from build123d import *

# Parameters (mm, degrees)
ESQUISSE1_W             = 260
ESQUISSE1_H             = 450
BOSS_EXTRU_1_DEPTH      = 130.18
ENL_V_MAT_EXTRU_1_REACH = 488.155
ESQUISSE2_W             = 240
ESQUISSE2_H             = 240.36


with BuildPart() as part:
    # Esquisse1 → Boss.-Extru.1 (new, symmetric)
    with BuildSketch(Plane.XY):
        Rectangle(ESQUISSE1_W, ESQUISSE1_H)
    extrude(amount=BOSS_EXTRU_1_DEPTH, both=True)

    # Esquisse2 → Enlèv. mat.-Extru.1 (cut, up to next)
    with BuildSketch(Plane(origin=(0, 225, 0), x_dir=(1, 0, 0), z_dir=(0, 1, 0)), mode=Mode.PRIVATE) as enl_v_mat_extru_1_sk1:
        Rectangle(ESQUISSE2_W, ESQUISSE2_H)
    enl_v_mat_extru_1_tool1 = extrude(enl_v_mat_extru_1_sk1.sketch, amount=-ENL_V_MAT_EXTRU_1_REACH, mode=Mode.PRIVATE) & part.part
    add(enl_v_mat_extru_1_tool1.solids().sort_by_distance((0, 225, 0))[0], mode=Mode.SUBTRACT)


solid = part.part
Here's how the part is built. I have some questions about the finished solid (model axes, mm). A direction names the side the tool comes from. Give positions to 0.01 mm unless a question says otherwise; leave off trailing zeros. Order: outer loops, then holes, each group sorted by start corner. A loop starts at its lowest first (then second) coordinate and runs counter-clockwise, first axis right, second up. Notation, with made-up numbers: M 88,-20.5 L 106,-20.5 A21 cw 106,-11.5 Z; hole C 41,54.5 d7. An arc over 180 degrees is marked long. Answer as a JSON object with one key per item and string values. Group by question number.
1) We'd pull the mould along Z, two halves only. Please class faces 3 (the flat face through (-2, 3, -120.18)), 4 (the flat face through (-2, 3, 130.18)), 5 (the flat face through (-10, -225, -125)): pulls with the +Z half, pulls with the -Z half, needs draft (parallel to the pull), parting line crosses it, or undercut.
2) Suppose I cut it at C-C, the plane y = -35.5. Write out the boundary of the cut face in (x, z).
3) Please list where these lines run through material, in increasing order: L1, parallel to Z at x = -3, y = -81.5; L2, parallel to X at y = 181, z = 78. Write a range as [from, to].
4) Suppose I cut it at A-A, the plane x = -77.5. Write out the boundary of the cut face in (y, z).
5) Suppose I cut it at B-B, the plane z = 79. Write out the boundary of the cut face in (x, y), plus the area to 3 significant figures.
6) On a 3-axis mill with a long thin cutter (end or side, diameter ignored), from which of +Z, -Z, +X, -X, +Y, -Y can I reach the whole of each face in a straight line? I mean faces 1 (the flat face through (-130, -3, 2)), 2 (the flat face through (-2, 3, 120.18)). Say none if no direction works.
Results found:
{
 "1": {"face 3": "undercut", "face 4": "pulls with the +Z half", "face 5": "needs draft"},
 "2": {"outline": "M -130,-130.18 L 130,-130.18 L 130,130.18 L -130,130.18 Z; hole M -120,-120.18 L 120,-120.18 L 120,120.18 L -120,120.18 Z"},
 "3": {"L1": "[-130.18, -120.18], [120.18, 130.18]", "L2": "[-130, -120], [120, 130]"},
 "4": {"outline": "M -225,-130.18 L 225,-130.18 L 225,-120.18 L -225,-120.18 Z; M -225,120.18 L 225,120.18 L 225,130.18 L -225,130.18 Z"},
 "5": {"outline": "M -130,-225 L -120,-225 L -120,225 L -130,225 Z; M 120,-225 L 130,-225 L 130,225 L 120,225 Z", "area": "9,000 mm²"},
 "6": {"face 1": "+Z, -Z, -X, +Y, -Y", "face 2": "+Y, -Y"}
}
